The figure shows three views and two pictorial views of one solid part (mm, origin at its lowest corner). Answer the questions. A direction names the side the tool comes from. Coordinates: 2 decimals unless noted, no trailing zeros. Write each loop counter-clockwise with the first axis right and the second up, starting at its lowest first coordinate (ties: lowest second). Pieces come first, ordered by that corner, then holes.
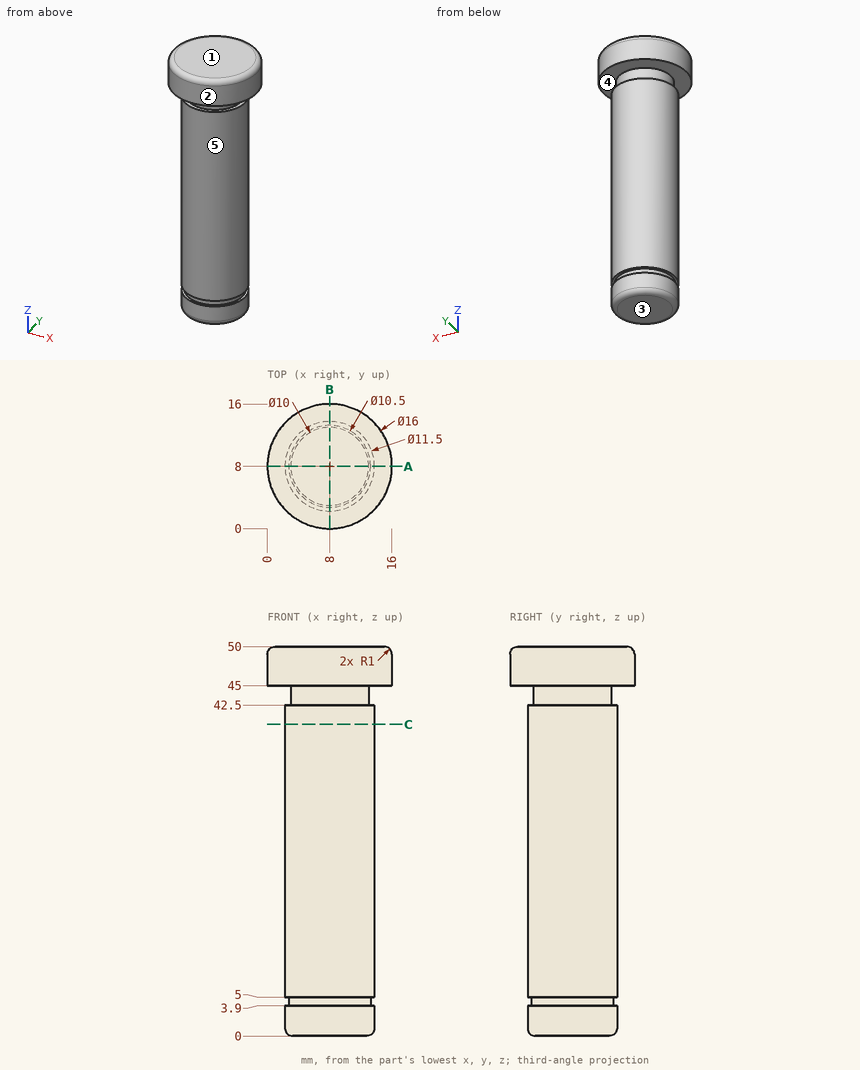
1. A tool of negligible diameter and unlimited length cuts with its end or side. For the marked faces 3, 4 and 5, from which of +Z, -Z, +X, -X, +Y, -Y can it reach the whole face along a straight path? Write none if from no direction.
Results found:
face 3: -Z, +X, -X, +Y, -Y
face 4: none
face 5: -Z
2. Section A-A on y = 8 is taken. Give the vertices of the cut face in (x, z), then the cut area to 3 significant figures.
Results found:
outline: (0, 45) - (3, 45) - (3, 42.5) - (2.25, 42.5) - (2.25, 5) - (2.75, 5) - (2.75, 3.9) - (2.25, 3.9) - (2.25, 1) arc R1 ccw to (3.25, 0) - (12.75, 0) arc R1 ccw to (13.75, 1) - (13.75, 3.9) - (13.25, 3.9) - (13.25, 5) - (13.75, 5) - (13.75, 42.5) - (13, 42.5) - (13, 45) - (16, 45) - (16, 49) arc R1 ccw to (15, 50) - (1, 50) arc R1 ccw to (0, 49) - close
area: 592 mm2
3. Section C-C on z = 40 is taken. Give the vertices of the cut face in (x, y), then the cut area to 3 significant figures.
Results found:
outline: circle Ø11.5 at (8, 8)
area: 104 mm2
4. Find the intervals of material crossed by L1, parallel to Z at x = 8, y = 13.5; L2, parallel to Z at x = 7.5, y = 1.75; L3, parallel to X at y = 7.75, z = 28, in increasing order.
Results found:
L1: z = 0.34 to 3.9, 5 to 42.5, 45 to 50
L2: z = 45 to 50
L3: x = 2.26 to 13.74
5. Flat-ended cylindrical pins translate along their axes: P1, Ø6, axis at x = 14.5, z = 30.5, coming from the +Y side; P2, Ø6, axis at x = 8, z = 34, coming from the -Y side; P3, Ø8, axis at y = 13, z = 25, coming from the +X side. Find the tip coordinate at first contact, or state that the pin passes through.
Results found:
P1: stops at y = 12.56
P2: stops at y = 2.25
P3: stops at x = 13.66
6. For a pull along X with two mould halves and no side action, classify the marked faces 1 and 2 as pulls with the +X half, pulls with the -X half, needs draft (parallel to the pull), parting line crosses it, or undercut.
Results found:
face 1: needs draft
face 2: parting line crosses it
